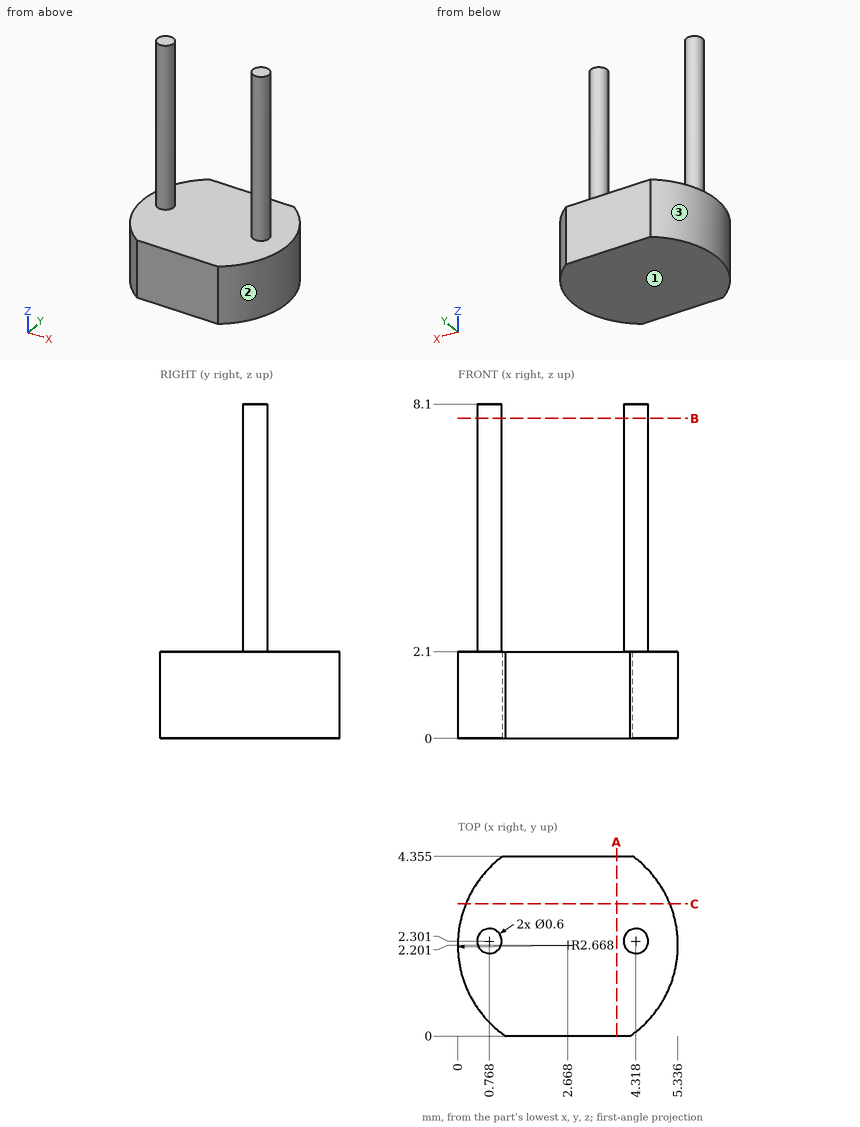
For this review, use the dimensioned drawing (mm, ordinates from the lowest corner) and the shaded views. Round coordinates to 2 decimals unless told otherwise and drop trailing zeros. Write each loop counter-clockwise with the first axis right and the second up, starting at its lowest first coordinate (ties: lowest second). Pieces come first, ordered by that corner, then holes. Notation, with made-up numbers: (-30, -10.5) - (-16, -10.5) arc R33 cw to (-16, 20.5) - close; hole circle Ø7 at (78.25, 88). An arc over 180 degrees is marked (long way). Answer as a JSON object with one key per item and string values.
1. We need section C-C on y = 3.2. Give the boundary of the cut face in (x, z) (1 decimal), then the cut area to 3 significant figures.
Response values:
{"outline": "(0.2, 0) - (5.1, 0) - (5.1, 2.1) - (0.2, 2.1) - close", "area": "10.4 mm2"}
2. We need section A-A on x = 3.85. Give the boundary of the cut face in (y, z) (1 decimal).
Response values:
{"outline": "(0, 0) - (4.4, 0) - (4.4, 2.1) - (0, 2.1) - close"}
3. For pin 1 Ø1 at (y, z) = (1, 4) entering from +X, flat-tipped, find the tip position at first contact; note if it passes through.
Response values:
{"pin 1": "passes through"}
4. To check wall thickness, follow line 1 along Z through (x, y) = (1.05, 0.5); line 2 along Y through (x, z) = (0.75, 6.5); line 3 along Y through (x, z) = (1.15, 2) (1 decimal). State the ranges of each line that lie inside material, in increasing order.
Response values:
{"line 1": "z = 0 to 2.1", "line 2": "y = 2 to 2.6", "line 3": "y = 0 to 4.4"}
5. Draft analysis for pull direction X (two halves, no side actions). For the marked faces 1, 2 and 3, state which applies: +X half, -X half, draft (parallel to the pull), parting line (faces both ways), or undercut.
Response values:
{"face 1": "draft", "face 2": "+X half", "face 3": "-X half"}
6. We need section B-B on z = 7.75. Give the boundary of the cut face in (x, y).
Response values:
{"outline": "circle Ø0.6 at (0.77, 2.3); circle Ø0.6 at (4.32, 2.3)"}
